Design review of the part built by this model. Coordinates are the model's own, in mm. Coordinates: 2 decimals unless noted, no trailing zeros. Order: outer loops, then holes, each group sorted by start corner. A loop starts at its lowest first (then second) coordinate and runs counter-clockwise, first axis right, second up.
from build123d import *

# Parameters (mm, degrees)
F0_W     = 263.652
F0_H     = 57.15
F1_DEPTH = 19.05
F2_W     = 6.7056
F2_H     = 15.24
F3_DEPTH = 6.35
F5_DEPTH = 6.35


with BuildPart() as f1:
    # F0 (on Right) → F1 (new body)
    with BuildSketch(Plane.YZ):
        Rectangle(F0_W, F0_H)
    extrude(amount=F1_DEPTH)

    # F2 (on face) → F3 (join)
    with BuildSketch(Plane.XZ.offset(131.826)):
        with Locations((9.7028, 7.493)):
            Rectangle(F2_W, F2_H)
    extrude(amount=F3_DEPTH)

    # F4 (on face) → F5 (join)
    with BuildSketch(Plane(origin=(0, 131.826, 0), x_dir=(-1, 0, 0), z_dir=(0, 1, 0))):
        Polygon((-6.35, 15.113), (-9.525, 15.113), (-13.0556, 15.113), (-13.0556, -0.127), (-6.35, -0.127), align=None)
    extrude(amount=F5_DEPTH)


solid = f1.part
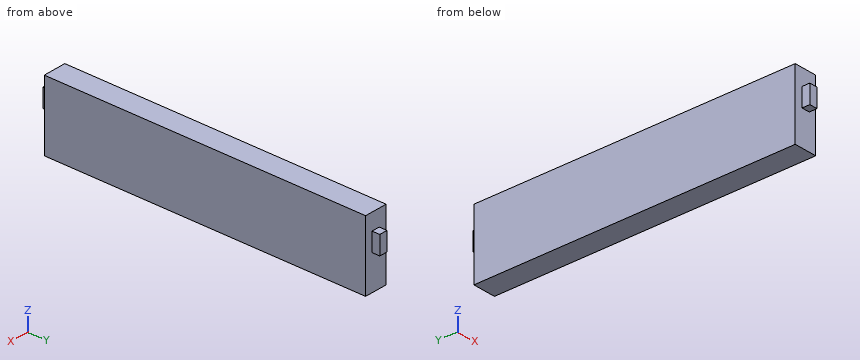
1. Add section A-A (z = 8). Give the boundary of the cut face in (x, y), and give its area (3 significant figures).
2. Add section B-B (x = 8.75). Give the boundary of the cut face in (y, z) (3 decimals), and give its area (3 significant figures).
3. To check wall thickness, follow line 1 (Y direction, x = 16, z = 21). State the ranges of the line that lie inside material, in increasing order.
4. Insertion check: pin 1 (3 mm diameter, centred on x = 7, z = -2, fed in from +Y); pin 2 (1.9 mm diameter, centred on x = 9.5, y = -136, fed in from -Z); pin 3 (5 mm diameter, centred on y = -136, z = 8, fed in from +X). Each pin has a flat end and moves straight along its axis. Give the tip position at first contact, or say it passes through.
Solution:
1. outline: (0, -131.83) - (6.35, -131.83) - (6.35, -138.18) - (13.06, -138.18) - (13.06, -131.83) - (19.05, -131.83) - (19.05, 131.83) - (13.06, 131.83) - (13.06, 138.18) - (6.35, 138.18) - (6.35, 131.83) - (0, 131.83) - close
1. area: 5,110 mm2
2. outline: (-138.176, -0.127) - (-131.826, -0.127) - (-131.826, -28.575) - (131.826, -28.575) - (131.826, -0.127) - (138.176, -0.127) - (138.176, 15.113) - (131.826, 15.113) - (131.826, 28.575) - (-131.826, 28.575) - (-131.826, 15.113) - (-138.176, 15.113) - close
2. area: 15,300 mm2
3. line 1: y = -131.83 to 131.83
4. pin 1: stops at y = 131.83
4. pin 2: stops at z = -0.13
4. pin 3: stops at x = 13.06
